from build123d import *

# Parameters (mm, degrees)
BOSS_EXTRUDE2_DEPTH      = 5.3975
SKETCH2_W                = 19.05
SKETCH2_H                = 13.716
CUT_EXTRUDE1_DEPTH       = 107.104395791
SKETCH3_R                = 38.1
CUT_EXTRUDE2_DEPTH       = 107.104395791
FILLET1_R                = 6.35
SKETCH8_R                = 1.651
CUT_EXTRUDE7_DEPTH       = 75.692
SKETCH10_R               = 1.651
CUT_EXTRUDE9_DEPTH       = 97.79
SKETCH11_R               = 1.651
CUT_EXTRUDE10_DEPTH      = 150.876
SKETCH12_R               = 3.175
CUT_EXTRUDE11_DEPTH      = 103.378
CUT_EXTRUDE11_DEPTH_BACK = 48.768
SKETCH13_R               = 6.35
CUT_EXTRUDE12_DEPTH      = 26.416


with BuildPart() as part:
    # Sketch1 → Boss-Extrude2 (new body)
    with BuildSketch(Plane.XY):
        with BuildLine():
            ThreePointArc((-69.525975721, 27.94), (-74.93, 0), (-69.525975721, -27.94))
            ThreePointArc((-69.525975721, -27.94), (0, -74.93), (69.525975721, -27.94))
            ThreePointArc((69.525975721, -27.94), (73.56658977, -14.228906128), (74.93, 0))
            ThreePointArc((74.93, 0), (73.56658977, 14.228906128), (69.525975721, 27.94))
            ThreePointArc((69.525975721, 27.94), (0, 74.93), (-69.525975721, 27.94))
        make_face()
        with BuildLine():
            ThreePointArc((-67.493975721, 26.416), (-67.122001333, 27.314025612), (-66.223975721, 27.686))
            Line((-66.223975721, 27.686), (-56.063975721, 27.686))
            Line((-56.063975721, 27.686), (-56.063975721, -27.686))
            Line((-56.063975721, -27.686), (-66.223975721, -27.686))
            ThreePointArc((-66.223975721, -27.686), (-67.122001333, -27.314025612), (-67.493975721, -26.416))
            Line((-67.493975721, -26.416), (-67.493975721, 26.416))
        make_face(mode=Mode.SUBTRACT)
        with BuildLine():
            ThreePointArc((66.223975721, 27.686), (67.122001333, 27.314025612), (67.493975721, 26.416))
            Line((67.493975721, 26.416), (67.493975721, -26.416))
            ThreePointArc((67.493975721, -26.416), (67.122001333, -27.314025612), (66.223975721, -27.686))
            Line((66.223975721, -27.686), (56.063975721, -27.686))
            Line((56.063975721, -27.686), (56.063975721, 27.686))
            Line((56.063975721, 27.686), (66.223975721, 27.686))
        make_face(mode=Mode.SUBTRACT)
    extrude(amount=BOSS_EXTRUDE2_DEPTH)

    # Sketch2 → Cut-Extrude1 (cut, through all)
    with BuildSketch(Plane.XY.offset(5.3975)):
        with Locations((0, 62.23)):
            Rectangle(SKETCH2_W, SKETCH2_H)
    extrude(amount=-CUT_EXTRUDE1_DEPTH, mode=Mode.SUBTRACT)

    # Sketch3 → Cut-Extrude2 (cut, through all)
    with BuildSketch(Plane.XY.offset(5.3975)):
        with Locations((0, -86.312058398)):
            Circle(SKETCH3_R)
    extrude(amount=-CUT_EXTRUDE2_DEPTH, mode=Mode.SUBTRACT)

    # Fillet1
    fillet1_edges = [part.edges().sort_by_distance(p)[0] for p in [
        (-33.000960548, -67.271401821, 2.69875),
        (33.000960548, -67.271401821, 2.69875),
    ]]
    fillet(fillet1_edges, radius=FILLET1_R)

    # Sketch8 → Cut-Extrude7 (cut)
    with BuildSketch(Plane(origin=(30.092005081, 4.08352975, -11.4935), x_dir=(-1, 0, 0), z_dir=(0, 0, -1))):
        with Locations(Location((63.757223581, 17.50647025, 0), (0, 0, 180))):
            Circle(SKETCH8_R)
        with Locations(Location((63.757223581, -25.67352975, 0), (0, 0, 180))):
            Circle(SKETCH8_R)
        with Locations(Location((-3.552776419, -25.67352975, 0), (0, 0, 180))):
            Circle(SKETCH8_R)
        with Locations(Location((-3.552776419, 17.50647025, 0), (0, 0, 180))):
            Circle(SKETCH8_R)
    extrude(amount=-CUT_EXTRUDE7_DEPTH, mode=Mode.SUBTRACT)

    # Sketch10 → Cut-Extrude9 (cut)
    with BuildSketch(Plane(origin=(30.092005081, 4.08352975, -41.529), x_dir=(-1, 0, 0), z_dir=(0, 0, -1))):
        with Locations(Location((4.154396091, -49.728759131, 0), (0, 0, 180))):
            Circle(SKETCH10_R)
        with Locations(Location((56.02961407, -49.728759131, 0), (0, 0, 180))):
            Circle(SKETCH10_R)
        with Locations(Location((4.154396091, 41.38247025, 0), (0, 0, 180))):
            Circle(SKETCH10_R)
        with Locations(Location((56.02961407, 41.38247025, 0), (0, 0, 180))):
            Circle(SKETCH10_R)
    extrude(amount=-CUT_EXTRUDE9_DEPTH, mode=Mode.SUBTRACT)

    # Sketch11 → Cut-Extrude10 (cut)
    with BuildSketch(Plane(origin=(30.092005081, 4.08352975, 5.3975), x_dir=(1, 0, 0), z_dir=(0, 0, 1))):
        with Locations((-101.395980802, -12.71952975)):
            Circle(SKETCH11_R)
        with Locations((-101.395980802, 4.55247025)):
            Circle(SKETCH11_R)
        with Locations((41.211970641, -12.71952975)):
            Circle(SKETCH11_R)
        with Locations((41.211970641, 4.55247025)):
            Circle(SKETCH11_R)
    extrude(amount=-CUT_EXTRUDE10_DEPTH, mode=Mode.SUBTRACT)

    # Sketch12 → Cut-Extrude11 (cut, two sides)
    with BuildSketch(Plane(origin=(30.092005081, 4.08352975, -5.3975), x_dir=(-1, 0, 0), z_dir=(0, 0, -1))) as cut_extrude11_sk:
        with Locations(Location((-16.897994919, 21.31647025, 0), (0, 0, 180))):
            Circle(SKETCH12_R)
        with Locations(Location((77.082005081, 21.31647025, 0), (0, 0, 180))):
            Circle(SKETCH12_R)
        with Locations(Location((30.092005081, 21.31647025, 0), (0, 0, 180))):
            Circle(SKETCH12_R)
        with Locations(Location((77.082005081, -29.48352975, 0), (0, 0, 180))):
            Circle(SKETCH12_R)
        with Locations(Location((30.092005081, -29.48352975, 0), (0, 0, 180))):
            Circle(SKETCH12_R)
        with Locations(Location((-16.897994919, -29.48352975, 0), (0, 0, 180))):
            Circle(SKETCH12_R)
    extrude(amount=CUT_EXTRUDE11_DEPTH, mode=Mode.SUBTRACT)
    extrude(cut_extrude11_sk.sketch, amount=-CUT_EXTRUDE11_DEPTH_BACK, mode=Mode.SUBTRACT)

    # Sketch13 → Cut-Extrude12 (cut)
    with BuildSketch(Plane(origin=(0, 0, 0), x_dir=(-1, 0, 0), z_dir=(0, 0, -1))):
        with Locations((46.99, 25.4)):
            Circle(SKETCH13_R)
        with Locations((0, 25.4)):
            Circle(SKETCH13_R)
        with Locations((-46.99, 25.4)):
            Circle(SKETCH13_R)
        with Locations((-46.99, -25.4)):
            Circle(SKETCH13_R)
        with Locations((0, -25.4)):
            Circle(SKETCH13_R)
        with Locations((46.99, -25.4)):
            Circle(SKETCH13_R)
    extrude(amount=-CUT_EXTRUDE12_DEPTH, mode=Mode.SUBTRACT)


solid = part.part
Design review of the part built by this model. Coordinates are the model's own, in mm. A direction names the side the tool comes from. Give positions to 0.01 mm unless a question says otherwise; leave off trailing zeros. Write each loop counter-clockwise with the first axis right and the second up, starting at its lowest first coordinate (ties: lowest second). Pieces come first, ordered by that corner, then holes. Notation, with made-up numbers: M 82.25,32.5 L 106.25,32.5 A22 cw 106.25,60.5 Z; hole C 46,-13.75 d2. An arc over 180 degrees is marked long. Answer as a JSON object with one key per item and string values. Group by question number.
1) Mouldability with a two-part tool opening along Y and no side actions: class faces 3 (the face through (0, 69.088, 3)), 4 (the face through (-1, 6, 5.398)) as released by +Y, released by -Y, zero draft, split by the parting line, or undercut.
2) Clearance check with flat-ended pins moving along their axes: pin 1 Ø7.5 at (x, y) = (0, 25.4) entering from -Z; pin 2 Ø1.6 at (x, z) = (60.5, 2.5) entering from +Y. State where each tip first meets the part, or that it passes through.
3) We need section B-B (x = -46). Give the boundary of the cut face in (y, z).
4) We need section C-C (y = 3). Give the boundary of the cut face in (x, z), and give its area (3 significant figures).
5) We need section A-A (y = -21.59). Count the separate pieces of the cut face and the enclosed holes in it, and give its area (3 significant figures).
6) For line 1 along X through (y, z) = (-1, 1.3); line 2 along X through (y, z) = (-19, 3.95); line 3 along Y through (x, z) = (-26, 0.7), list the stretches that pass through material, from the lowest coordinate up.
7) Tool access review of faces 1 (the face through (-1, 6, 0)), 2 (the face through (56.064, 0, 3)): name each direction out of +Z, -Z, +X, -X, +Y, -Y from which nothing blocks a thin tool from reaching the whole face with its end or side.
Answer key:
{
 "1": {"face 3": "undercut", "face 4": "zero draft"},
 "2": {"pin 1": "passes through", "pin 2": "stops at y = 45.28"},
 "3": {"outline": "M -59.15,0 L -31.67,0 L -31.67,5.4 L -59.15,5.4 Z; M -19.13,0 L 19.13,0 L 19.13,5.4 L -19.13,5.4 Z; M 31.67,0 L 59.15,0 L 59.15,5.4 L 31.67,5.4 Z"},
 "4": {"outline": "M -74.87,0 L -67.49,0 L -67.49,5.4 L -74.87,5.4 Z; M -56.06,0 L 56.06,0 L 56.06,5.4 L -56.06,5.4 Z; M 67.49,0 L 74.87,0 L 74.87,5.4 L 67.49,5.4 Z", "area": "685 mm²"},
 "5": {"separate pieces": "8", "enclosed holes": "0", "area": "451 mm²"},
 "6": {"line 1": "x = -74.92 to -67.49, -56.06 to 56.06, 67.49 to 74.92", "line 2": "x = -72.48 to -67.49, -56.06 to 56.06, 67.49 to 72.48", "line 3": "y = -58.46 to -47.3, -44 to 43.82, 47.12 to 70.27"},
 "7": {"face 1": "-Z, +X, -X, +Y, -Y", "face 2": "+Z, -Z"}
}
